The listing builds one solid part. Answer for the finished solid, in the listing's coordinates (mm). A direction names the side the tool comes from. Coordinates: 2 decimals unless noted, no trailing zeros. Loops run counter-clockwise (first coordinate to the right, second up) from the corner with the lowest first, then second, coordinate; pieces in that order, holes last. Notation, with made-up numbers: M 66,37.5 L 108,37.5 A16 cw 108,53.5 Z; hole C -20.75,-25.75 d7. An arc over 180 degrees is marked long. Return JSON: item names as keys, results as strings. Group by question number.
1. Which of the six approach directions +Z, -Z, +X, -X, +Y, -Y give full straight-line access (tool end or side, diameter ignored) to faces 4 (the face through (-34, 12, 16)), 5 (the face through (-8.468, -18.237, 3.695)), 6 (the face through (-83.703, -17, 11))?
2. Section A-A (z = 0) is taken. Write down the section's boundary in (x, y), then the cut area to 3 significant figures.
3. Straight lines are drawn through the part: L1, parallel to X at y = 17.85, z = 0; L2, parallel to X at y = -8.5, z = -6; L3, parallel to Y at x = -38, z = 0. For each, find the intervals that lie inside material, in ascending order. Write a range as from..to.
4. Section D-D (y = -7) is taken. Count the separate pieces of the cut face and the enclosed holes in it, then the cut area to 3 significant figures.
5. The mould has two halves that part along X. Classify faces 1 (the face through (-66.784, -17, -11)), 2 (the face through (-94.62, -0.88, 19.98)), 3 (the face through (-8.47, 16.93, 7.73)): pulls with the +X half, pulls with the -X half, needs draft (parallel to the pull), parting line crosses it, or undercut.
6. Given P1, Ø10, axis at y = -5, z = -6.5, coming from the -X side; P2, Ø10.5, axis at x = -10, z = 0, coming from the -Y side; P3, Ø1.5, axis at x = -30, z = -18, coming from the -Y side, each flat-ended and moving along its own axis, determine where each tip first touches the part or whether it passes through.
7. Section C-C (x = -90) is taken. Write down the section's boundary in (y, z).
8. Section B-B (y = 0) is taken. Write down the section's boundary in (x, z).
```python
from build123d import *

# Parameters (mm, degrees)
CUT_EXTRUDE1_REACH      = 113.025
CUT_EXTRUDE1_END_RADIUS = 20
SKETCH2_R               = 4
CIRPATTERN1_COUNT       = 10


with BuildPart() as part:
    # Sketch1 → Revolve1 (revolve)
    with BuildSketch(Plane.XY, mode=Mode.PRIVATE) as revolve1_sk:
        Polygon((0, 0), (0, 20), (-66.784359743, 20), (-66.784359743, 25), (-83.702975636, 25), (-83.702975636, 20), (-105.24487755, 20), (-105.24487755, 17), (-3, 17), (-3, 0), align=None)
    revolve(revolve1_sk.sketch.rotate(Axis((27.57498519, 0, 0), (-1, 0, 0)), 90), axis=Axis((27.57498519, 0, 0), (-1, 0, 0)))

    # Cut-Extrude1: up to this cylinder (the profile starts inside it)
    cut_extrude1_end = Plane(origin=(-10, 0, 0), z_dir=(1, 0, 0)) * Cylinder(CUT_EXTRUDE1_END_RADIUS, 267.05, mode=Mode.PRIVATE)
    # Sketch2 → Cut-Extrude1 (cut, up to the surface)
    with BuildSketch(Plane(origin=(0, 0, 0), x_dir=(1, 0, 0), z_dir=(0, 1, 0)), mode=Mode.PRIVATE) as cut_extrude1_sk1:
        with Locations(Location((-10, 0, 0), (0, 0, 90))):
            Circle(SKETCH2_R)
    cut_extrude1_tool1 = extrude(cut_extrude1_sk1.sketch, amount=CUT_EXTRUDE1_REACH, mode=Mode.PRIVATE) & cut_extrude1_end
    cut_extrude1 = cut_extrude1_tool1.solids().sort_by_distance((-10, 0, 0))[0]
    add(cut_extrude1, mode=Mode.SUBTRACT)

    # CirPattern1: Cut-Extrude1 ×10 about axis
    cirpattern1_axis = Axis((27.57498519, 0, 0), (-1, 0, 0))
    for i in range(1, CIRPATTERN1_COUNT):
        add(cut_extrude1.rotate(cirpattern1_axis, i * 360 / CIRPATTERN1_COUNT), mode=Mode.SUBTRACT)


solid = part.part
```
Worked out:
{
 "1": {"face 4": "+X", "face 5": "+Y, -Y", "face 6": "-X"},
 "2": {"outline": "M -105.24,-20 L -83.7,-20 L -83.7,-25 L -66.78,-25 L -66.78,-20 L -14,-20 L -14,-17 L -105.24,-17 Z; M -105.24,17 L -14,17 L -14,20 L -66.78,20 L -66.78,25 L -83.7,25 L -83.7,20 L -105.24,20 Z; M -6,-20 L 0,-20 L 0,20 L -6,20 L -6,17 L -3,17 L -3,-17 L -6,-17 Z", "area": "855 mm^2"},
 "3": {"L1": "-105.24..-14, -6..0", "L2": "-3..0", "L3": "-20..-17, 17..20"},
 "4": {"separate pieces": "3", "enclosed holes": "0", "area": "905 mm^2"},
 "5": {"face 1": "pulls with the +X half", "face 2": "needs draft", "face 3": "undercut"},
 "6": {"P1": "x = -3", "P2": "y = -20", "P3": "y = -10.12"},
 "7": {"outline": "C 0,0 d40; hole C 0,0 d34"},
 "8": {"outline": "M -105.24,-20 L -83.7,-20 L -83.7,-25 L -66.78,-25 L -66.78,-20 L 0,-20 L 0,20 L -66.78,20 L -66.78,25 L -83.7,25 L -83.7,20 L -105.24,20 L -105.24,17 L -3,17 L -3,-17 L -105.24,-17 Z"}
}
